Autodesk Inventor part; units mm, degrees
ref_plane "YZ Plane" through (0, 0, 0) normal (1, 0, 0) x (0, 1, 0)
ref_plane "XZ Plane" through (0, 0, 0) normal (0, 1, 0) x (-1, 0, 0)
ref_plane "XY Plane" through (0, 0, 0) normal (0, 0, 1) x (1, 0, 0)
sketch "Sketch1" plane through (0, 0, 0) normal (1, 0, 0) x (0, 1, 0)
  line L0 (0, 0) -> (30, 0)
  line L1 (30, 0) -> (30, -160)
  line L2 (30, -160) -> (0, -160)
  line L3 (0, -160) -> (0, 0)
  line L4 (25, -20) -> (5, -20)
  line L5 (0, -20) -> (0, -25)
  line L6 (5, -25) -> (25, -25)
  line L7 (30, -25) -> (30, -20)
  line L8 (25, -35) -> (5, -35)
  line L9 (0, -35) -> (0, -40)
  line L10 (5, -40) -> (25, -40)
  line L11 (30, -40) -> (30, -35)
  line L12 (25, -50) -> (5, -50)
  line L13 (0, -50) -> (0, -55)
  line L14 (5, -55) -> (25, -55)
  line L15 (30, -55) -> (30, -50)
  line L16 (25, -75) -> (5, -75)
  line L17 (0, -75) -> (0, -85)
  line L18 (5, -85) -> (25, -85)
  line L19 (30, -85) -> (30, -75)
  line L20 (25, -105) -> (5, -105)
  line L21 (0, -105) -> (0, -110)
  line L22 (5, -110) -> (25, -110)
  line L23 (30, -110) -> (30, -105)
  line L24 (25, -120) -> (5, -120)
  line L25 (0, -120) -> (0, -125)
  line L26 (5, -125) -> (25, -125)
  line L27 (30, -125) -> (30, -120)
  line L28 (25, -135) -> (5, -135)
  line L29 (0, -135) -> (0, -140)
  line L30 (5, -140) -> (25, -140)
  line L31 (30, -140) -> (30, -135)
  line L32 (30, 0) -> (25, 0)
  line L33 (25, 0) -> (25, -160)
  line L34 (25, -160) -> (30, -160)
  line L35 (30, -160) -> (30, 0)
  line L36 (0, 0) -> (5, 0)
  line L37 (5, 0) -> (5, -160)
  line L38 (5, -160) -> (0, -160)
  line L39 (0, -160) -> (0, 0)
  line L40 (30, 0) -> (0, 0)
  line L41 (0, 0) -> (0, 5)
  line L42 (0, 5) -> (30, 5)
  line L43 (30, 5) -> (30, 0)
  line L44 (30, -160) -> (0, -160)
  line L45 (0, -160) -> (0, -165)
  line L46 (0, -165) -> (30, -165)
  line L47 (30, -165) -> (30, -160)
  dimension "d0" = 30
  dimension "d1" = 160
  dimension "d2" = 5
  dimension "d3" = 20
  dimension "d4" = 5
  dimension "d5" = 5
  dimension "d6" = 10
  dimension "d7" = 5
  dimension "d8" = 5
  dimension "d9" = 5
  dimension "d10" = 20
  dimension "d12" = 10
  dimension "d14" = 20
  dimension "d15" = 10
  dimension "d16" = 10
  dimension "d17" = 10
  dimension "d18" = 5
  dimension "d19" = 5
  dimension "d20" = 5
  dimension "d21" = 5
extrude "Extrusion1" add sketch "Sketch1" along normal blind 10 contours L0 L37 L2 L3 | L0 L33 L4 L37 | L0 L1 L2 L33 | L6 L33 L8 L37 | L10 L33 L12 L37 | L14 L33 L16 L37 | L18 L33 L20 L37 | L22 L33 L24 L37 | L26 L33 L28 L37 | L30 L33 L2 L37
extrude "Extrusion2" add sketch "Sketch1" along normal blind 80 contours L41 L42 L43 L0 | L2 L47 L46 L45
sketch "Sketch2" plane through (0, 0, 5) normal (0, 0, 1) x (1, 0, 0)
  line L0 (80, 30) -> (80, 0)
  line L1 (0, 0) -> (80, 0)
  point P0 (75, 25)
  dimension "d33" = 5
  dimension "d34" = 25
hole "Hole1" at (75, 25, 5) direction (0, 0, -1) diameter 3 end through all
properties part number "BONNET"
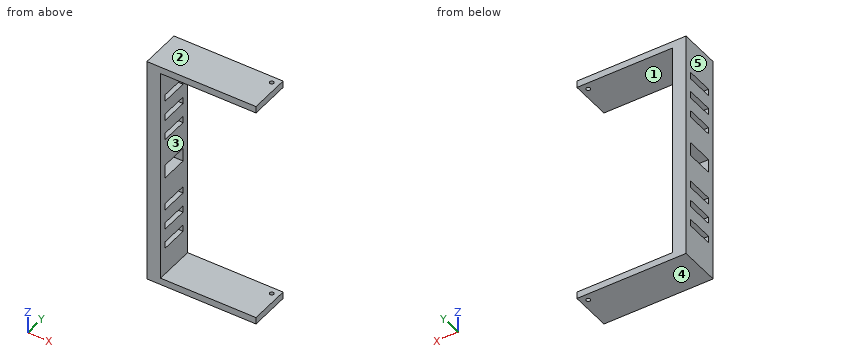
Model file for the job. Use its own axes, mm. Face numbers are marked on the shaded views. A direction names the side the tool comes from. Round coordinates to 2 decimals unless told otherwise and drop trailing zeros. Loops run counter-clockwise (first coordinate to the right, second up) from the corner with the lowest first, then second, coordinate; pieces in that order, holes last. Notation, with made-up numbers: M 64.25,11.25 L 120.25,11.25 A21 ccw 120.25,36.25 Z; hole C 36.5,-19 d10. An arc over 180 degrees is marked long. Put each result on its own line as item: value. Start each with the question number.
Item 1: Mould opens along Z. For the marked faces 3, 4 and 5 say: released by +Z, released by -Z, zero draft, split by the parting line, or undercut.
Item 2: Cut at C-C (z = -129). List the corners of the cut face in (x, y).
Item 3: 3-axis set-ups, long thin cutter, end or side, ignore diameter. For the marked faces 1 and 2: which of +Z, -Z, +X, -X, +Y, -Y reach the whole face in a straight line?
Item 4: Drill centre lines: line 1 along Z through (x, y) = (63.5, 11.5); line 2 along Y through (x, z) = (75, 2); line 3 along X through (y, z) = (25, 3.6). Where is each one in solid material? Low to high.
Item 5: Cut at B-B (x = 6). Give the number of separate pieces and of enclosed holes in the cut face, then the cut area to 3 significant figures.
Item 6: Drop a flat-ended pin along its axis: P1, Ø3, axis at y = 8, z = -85, coming from the +X side. Give the stop position or say it passes through.
Item 7: Cut at A-A (x = 59.5). List the corners of the cut face in (y, z), then the cut area to 3 significant figures.
Answer block:
1. face 3: undercut
1. face 4: released by -Z
1. face 5: zero draft
2. outline: M 0,0 L 10,0 L 10,30 L 0,30 Z
3. face 1: +X, +Y, -Y
3. face 2: +Z, +X, -X, +Y, -Y
4. line 1: -165 to -160, 0 to 5
4. line 2: 0 to 23.5, 26.5 to 30
4. line 3: 0 to 73.5, 76.5 to 80
5. separate pieces: 1
5. enclosed holes: 7
5. area: 4,300 mm2
6. P1: x = 10
7. outline: M 0,-165 L 30,-165 L 30,-160 L 0,-160 Z; M 0,0 L 30,0 L 30,5 L 0,5 Z
7. area: 300 mm2
